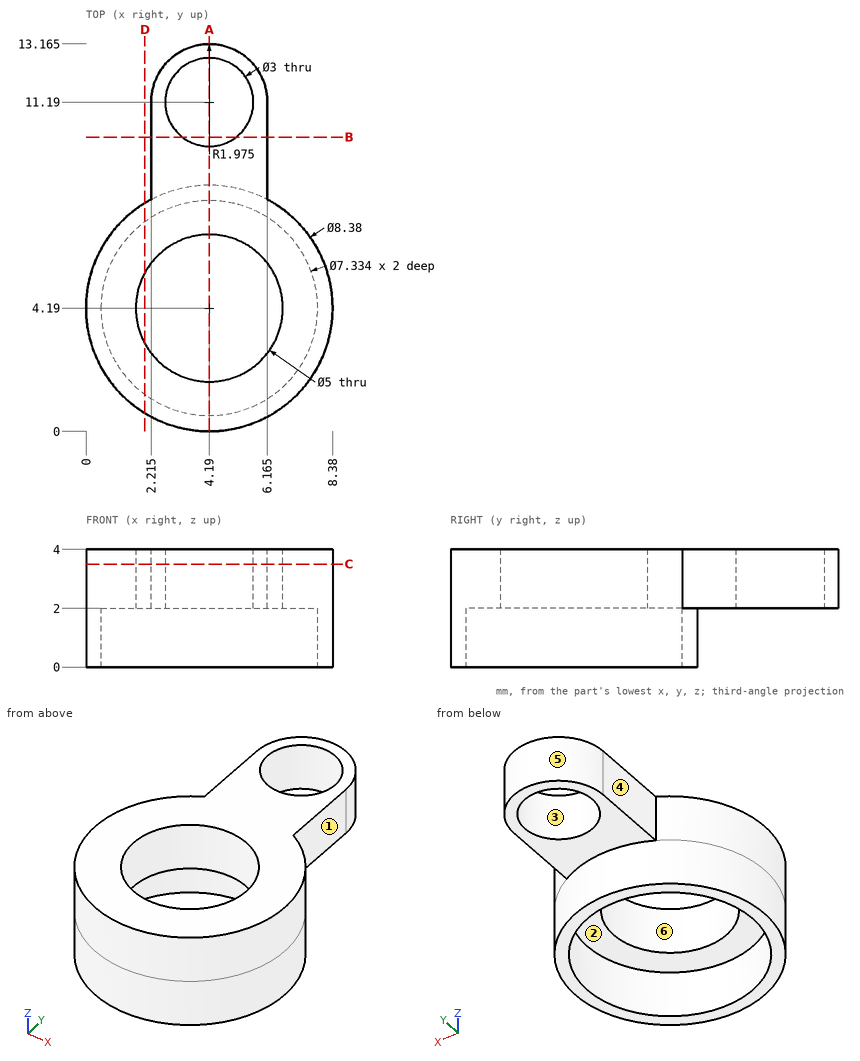
Check sheet for the drawn part. Datum: minimum x, y, z corner. Units: mm. A direction names the side the tool comes from. Give positions to 0.01 mm unless a question says otherwise; leave off trailing zeros. Order: outer loops, then holes, each group sorted by start corner. A loop starts at its lowest first (then second) coordinate and runs counter-clockwise, first axis right, second up. Notation, with made-up numbers: (-23, -3.5) - (26, -3.5) arc R22 ccw to (26, 26.5) - close; hole circle Ø11 at (8.25, -19.5). An arc over 180 degrees is marked (long way). Answer as a JSON object with one key per item and string values.
(1) Tool access check on the marked faces 1, 2 and 3. Record the directions out of +Z, -Z, +X, -X, +Y, -Y that give a thin tool (end or side, any length) a straight path to the whole face; none if there is none.
Report:
{"face 1": "+Z, -Z, +X, +Y", "face 2": "-Z", "face 3": "+Z, -Z"}
(2) Cross-section at D-D (x = 2). Record the cut outline in (y, z).
Report:
{"outline": "(0.62, 0) - (1.25, 0) - (1.25, 2) - (2.98, 2) - (2.98, 4) - (0.62, 4) - close; (5.4, 2) - (7.13, 2) - (7.13, 0) - (7.76, 0) - (7.76, 4) - (5.4, 4) - close"}
(3) Draft check along X on the marked faces 4, 5 and 6. Enter one of: released by +X, released by -X, zero draft, split by the parting line, or undercut.
Report:
{"face 4": "released by -X", "face 5": "split by the parting line", "face 6": "undercut"}
(4) Cross-section at C-C (z = 3.5). State how many separate pieces and enclosed holes the cut face has, then the cut area to 3 significant figures.
Report:
{"separate pieces": "1", "enclosed holes": "2", "area": "46.3 mm^2"}
(5) Cross-section at B-B (y = 10). Record the cut outline in (x, z) (1 decimal).
Report:
{"outline": "(2.2, 2) - (3.3, 2) - (3.3, 4) - (2.2, 4) - close; (5.1, 2) - (6.2, 2) - (6.2, 4) - (5.1, 4) - close"}
(6) Material ranges on line 1 (Y direction, x = 4.19, z = 3.5) (1 decimal); line 2 (Y direction, x = 4.19, z = 0.9); line 3 (Y direction, x = 3.25, z = 2.95) (1 decimal), recorded low to high.
Report:
{"line 1": "0 to 1.7, 6.7 to 9.7, 12.7 to 13.2", "line 2": "0 to 0.52, 7.86 to 8.38", "line 3": "0.1 to 1.9, 6.5 to 10, 12.4 to 12.9"}
(7) Cross-section at A-A (x = 4.19). Record the cut outline in (y, z) (1 decimal).
Report:
{"outline": "(0, 0) - (0.5, 0) - (0.5, 2) - (1.7, 2) - (1.7, 4) - (0, 4) - close; (6.7, 2) - (7.9, 2) - (7.9, 0) - (8.4, 0) - (8.4, 2) - (9.7, 2) - (9.7, 4) - (6.7, 4) - close; (12.7, 2) - (13.2, 2) - (13.2, 4) - (12.7, 4) - close"}
(8) Depth check by flat-ended pin: pin 1 Ø1 at (x, z) = (6, 3.5) entering from -Y; pin 2 Ø1.6 at (y, z) = (9.5, 3) entering from -X (3 decimals); pin 3 Ø1 at (y, z) = (10.5, 2.5) entering from +X (3 decimals). Enter the tip coordinate at first touch or a pass-through.
Report:
{"pin 1": "y = 0.21", "pin 2": "x = 2.215", "pin 3": "x = 6.165"}
